Work out the finished part from the listing and answer in its coordinate system (mm). A direction names the side the tool comes from. Coordinates: 2 decimals unless noted, no trailing zeros. Loops run counter-clockwise (first coordinate to the right, second up) from the corner with the lowest first, then second, coordinate; pieces in that order, holes last. Notation, with made-up numbers: (12.25, -23.5) - (45.25, -23.5) arc R20 ccw to (45.25, -19.5) - close; hole circle Ø9 at (-25.75, 80). An arc over 180 degrees is marked (long way). Write each question's results on one line, items separated by ' | '. Start each with the question number.
Item 1: Consider probe 1 along Z at (x, y) = (219, 287); probe 2 along Y at (x, z) = (212, 546); probe 3 along Y at (x, z) = (30.5, 506). Determine where each line is inside the solid, lowest interval first. Write a range as [from, to].
Item 2: Section B-B, the plane x = 248.5 is taken. Write down the section's boundary in (y, z), plus the area to 3 significant figures.
Item 3: Section A-A, the plane z = 524.5 is taken. Write down the section's boundary in (x, y), plus the area to 3 significant figures.
Item 4: A tool of negligible diameter and unlimited length cuts with its end or side. For faces 5 (the face through (197, 197, 0)), 6 (the face through (175, 285, 525)), 7 (the face through (202.8, 150, 582.4)), from which of +Z, -Z, +X, -X, +Y, -Y can it reach the whole face along a straight path? Write none if from no direction.
Item 5: Section C-C, the plane x = 77 is taken. Write down the section's boundary in (y, z), plus the area to 3 significant figures.
Item 6: Each of these flat-tipped pins is pushed along its axis until it touches: pin 1 Ø2 at (x, y) = (165, 153.5) entering from +Z; pin 2 Ø3 at (x, z) = (196.5, 367) entering from -Y. Where does it stop, or does it pass through?
Item 7: For a pull along Y with two mould halves and no side action, classify faces 1 (the face through (197, 0, 296)), 2 (the face through (197, 400, 296)), 3 (the face through (197, 334, 600)), 4 (the face through (200, 300, 525)) as +Y half, -Y half, draft (parallel to the pull), parting line (faces both ways), or undercut.
Item 8: Section D-D, the plane y = 216 is taken. Write down the section's boundary in (x, z), plus the area to 3 significant figures.
from build123d import *

# Parameters (mm, degrees)
F0_W        = 400
F0_H        = 600
F1_DEPTH    = 200
F2_W        = 30
F2_H        = 50
F3_DEPTH    = 25
F1_FACE_W   = 400
F1_FACE_H   = 600
F1_FACE_W_2 = 30
F1_FACE_H_2 = 50
F4_DEPTH    = 25
F5_W        = 400
F5_H        = 600
F6_DEPTH    = 175
F8_DEPTH    = 400.001
F9_W        = 184
F9_H        = 92
F10_DEPTH   = 1


with BuildPart() as f1:
    # F0 (on Right) → F1 (new body)
    with BuildSketch(Plane.YZ):
        with Locations((200, 300)):
            Rectangle(F0_W, F0_H)
    extrude(amount=F1_DEPTH)

    # F2 (on face) → F3 (cut)
    with BuildSketch(Plane.YZ.offset(200)):
        with Locations((285, 525)):
            Rectangle(F2_W, F2_H)
    extrude(amount=-F3_DEPTH, mode=Mode.SUBTRACT)

    # F1_face (on face) → F4 (join)
    with BuildSketch(Plane(origin=(200, 200, 300), x_dir=(0, 1, 0), z_dir=(1, 0, 0))):
        Rectangle(F1_FACE_W, F1_FACE_H)
        with Locations((85, 225)):
            Rectangle(F1_FACE_W_2, F1_FACE_H_2, mode=Mode.SUBTRACT)
    extrude(amount=F4_DEPTH)

    # F5 (on face) → F6 (join)
    with BuildSketch(Plane.YZ.offset(225)):
        with Locations((200, 300)):
            Rectangle(F5_W, F5_H)
    extrude(amount=F6_DEPTH)

    # F7 (on face) → F8 (cut, through all)
    with BuildSketch(Plane.YZ.offset(400)):
        Polygon((270, 550), (270, 600), (150, 600), (150, 490), (270, 490), (270, 500), align=None)
    extrude(amount=-F8_DEPTH, mode=Mode.SUBTRACT)

    # F9 (on face) → F10 (cut)
    with BuildSketch(Plane(origin=(0, 150, 0), x_dir=(-1, 0, 0), z_dir=(0, 1, 0))):
        with Locations((-200, 536)):
            Rectangle(F9_W, F9_H)
    extrude(amount=-F10_DEPTH, mode=Mode.SUBTRACT)


solid = f1.part
Answer key:
1) probe 1: z = [0, 500], [550, 600] | probe 2: y = [0, 149], [300, 400] | probe 3: y = [0, 150], [270, 400]
2) outline: (0, 0) - (400, 0) - (400, 600) - (270, 600) - (270, 490) - (149, 490) - (149, 582) - (150, 582) - (150, 600) - (0, 600) - close | area: 227,000 mm^2
3) outline: (0, 0) - (400, 0) - (400, 150) - (292, 150) - (292, 149) - (108, 149) - (108, 150) - (0, 150) - close; (0, 270) - (175, 270) - (175, 300) - (225, 300) - (225, 270) - (400, 270) - (400, 400) - (0, 400) - close | area: 110,000 mm^2
4) face 5: -Z, +X, -X, +Y, -Y | face 6: none | face 7: +Z, +X, -X
5) outline: (0, 0) - (400, 0) - (400, 600) - (270, 600) - (270, 490) - (150, 490) - (150, 600) - (0, 600) - close | area: 227,000 mm^2
6) pin 1: stops at z = 490 | pin 2: stops at y = 0
7) face 1: -Y half | face 2: +Y half | face 3: draft | face 4: undercut
8) outline: (0, 0) - (400, 0) - (400, 490) - (0, 490) - close | area: 196,000 mm^2
